Check sheet for the modelled part. Datum: model origin and axes. Units: mm. A direction names the side the tool comes from. Round coordinates to 2 decimals unless told otherwise and drop trailing zeros. Order: outer loops, then holes, each group sorted by start corner. A loop starts at its lowest first (then second) coordinate and runs counter-clockwise, first axis right, second up. Notation, with made-up numbers: (9.5, 14.5) -> (53.5, 14.5) arc R22 cw to (53.5, 50.5) -> close; hole circle Ø1 at (86.5, 3.25). An arc over 180 degrees is marked (long way). Answer in a Markdown table with one row per item. Add a question column.
1. Depth check by flat-ended pin: P1, Ø5, axis at y = 186.5, z = -7, coming from the -X side; P2, Ø8, axis at y = 203.5, z = -3, coming from the -X side; P3, Ø5, axis at y = 207, z = -0.5, coming from the +X side. Enter the tip coordinate at first touch or a pass-through.
2. Sectioned sample at B-B, the plane z = -7.25. Record the boundary of the cut face in (x, y).
3. Sectioned sample at A-A, the plane y = 211. Record the boundary of the cut face in (x, z) (3 decimals), then the cut area to 3 significant figures.
4. Access from +Z, -Z, +X, -X, +Y, -Y to the whole of each face (thin tool, end or side, straight path). Record for faces 1 (the flat face through (-13, 228, 3.175)), 2 (the flat face through (-72, 215, -9.525)).
5. Sectioned sample at C-C, the plane x = -35. Record the boundary of the cut face in (y, z) (3 decimals).
6. Material ranges on L1, parallel to Z at x = -16, y = 214.5 (3 decimals); L2, parallel to X at y = 188.5, z = -6; L3, parallel to Y at x = -114.5, z = 6.5, recorded low to high. Write a range as from..to.
7. Sectioned sample at D-D, the plane y = 240.5. Record the boundary of the cut face in (x, z) (3 decimals), then the cut area to 3 significant figures.
```python
from build123d import *

# Parameters (mm, degrees)
F1_DEPTH = 9.525
F3_DEPTH = 12.7


with BuildPart() as f1:
    # F0 (on Top) → F1 (new body, symmetric)
    with BuildSketch(Plane.XY):
        with BuildLine():
            Line((-7.5431177714, 203.059945273), (-9.4288972142, 253.8249315913))
            ThreePointArc((-9.4288972142, 253.8249315913), (-69.899192714, 244.192757587), (-126.3072012065, 220.3689881162))
            Line((-126.3072012065, 220.3689881162), (-101.0457609652, 176.295190493))
            ThreePointArc((-101.0457609652, 176.295190493), (-55.9193541712, 195.3542060696), (-7.5431177714, 203.059945273))
        make_face()
    extrude(amount=F1_DEPTH, both=True)

    # F2 (on face) → F3 (cut)
    with BuildSketch(Plane(origin=(0, 0, -9.525), x_dir=(1, 0, 0), z_dir=(0, 0, -1))):
        with BuildLine():
            ThreePointArc((-7.5431177714, -203.059945273), (-12.3015704517, -202.8272944266), (-17.0532610321, -202.4831506278))
            Line((-17.0532610321, -202.4831506278), (-18.9407001232, -253.292814503))
            ThreePointArc((-18.9407001232, -253.292814503), (-14.1872936257, -253.6034713871), (-9.4288972142, -253.8249315913))
            Line((-9.4288972142, -253.8249315913), (-7.5431177714, -203.059945273))
        make_face()
    extrude(amount=-F3_DEPTH, mode=Mode.SUBTRACT)


solid = f1.part
```
Answer key:
| question | item | result |
|---|---|---|
| 1 | P1 | stops at x = -108.33 |
| 1 | P2 | stops at x = -118.93 |
| 1 | P3 | stops at x = -17.13 |
| 2 | outline | (-126.31, 220.37) -> (-101.05, 176.3) arc R203.2 cw to (-17.05, 202.48) -> (-18.94, 253.29) arc R254 ccw to start |
| 3 | outline | (-120.937, -9.525) -> (-17.37, -9.525) -> (-17.37, 3.175) -> (-7.838, 3.175) -> (-7.838, 9.525) -> (-120.937, 9.525) -> close |
| 3 | area | 2,030 mm² |
| 4 | face 1 | -Z, +X, +Y |
| 4 | face 2 | -Z, +X, -X, +Y, -Y |
| 5 | outline | (200.163, -9.525) -> (251.577, -9.525) -> (251.577, 9.525) -> (200.163, 9.525) -> close |
| 6 | L1 | z = 3.175..9.525 |
| 6 | L2 | x = -108.04..-75.88 |
| 6 | L3 | y = 199.77..226.73 |
| 7 | outline | (-81.705, -9.525) -> (-18.465, -9.525) -> (-18.465, 3.175) -> (-8.934, 3.175) -> (-8.934, 9.525) -> (-81.705, 9.525) -> close |
| 7 | area | 1,270 mm² |
